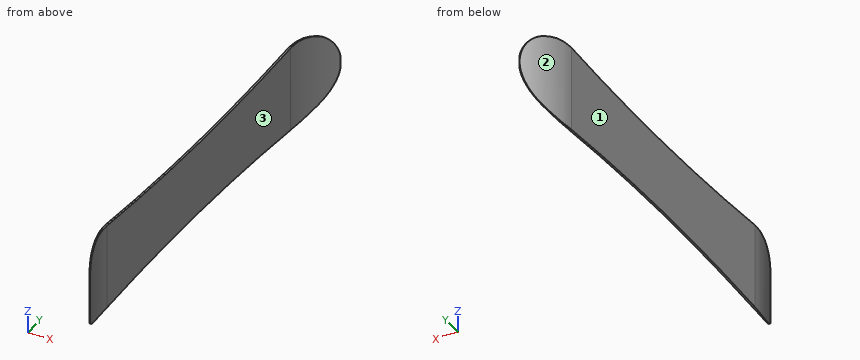
Solid Edge part; units mm, degrees
sketch "Sketch1" plane through (0, 0, 0) normal (1, 0, 0) x (0, 1, 0)
  arc A0 (-585.5098, 151.2) -> (585.5098, 151.2) centre (0, 7528) ccw
  line L0 (585.5098, 151.2) -> (585.5098, -151.2)
  arc A1 (-585.5098, -151.2) -> (585.5098, -151.2) centre (0, -7528) cw
  line L1 (-585.5098, 151.2) -> (-585.5098, -151.2)
extrude "Protrusion1" add sketch "Sketch1" against normal blind 7
sketch "Sketch2" plane through (0, -800, 0) normal (0, 0, -1) x (1, 0, 0)
  arc A0 (59.1552, -1.148) -> (0, -214.4902) centre (414.2845, -214.4902) ccw
  line L0 (0, -214.4902) -> (-7, -214.4902)
  arc A1 (-7, -214.4902) -> (57.4408, -0.1181) centre (446.8281, -234.0406) cw
  line L1 (57.4408, -0.1181) -> (59.1552, -1.148)
extrude "ExtrudedProtrusion_4" add sketch "Sketch2" along normal mid plane 302.4
sketch "Sketch3" plane through (59.1552, 0, 0) normal (1, 0, 0) x (0, 0, 1)
  arc A0 (-128, 717.5098) -> (128, 717.5098) centre (0, 659.2447) cw
  arc A1 (128, 717.5098) -> (151.2, 585.5098) centre (-115.4835, 606.677) cw
  line L0 (265.9453, 585.5098) -> (151.2, 585.5098)
  line L1 (265.9453, 882.5583) -> (265.9453, 585.5098)
  line L2 (-248.3835, 882.5583) -> (265.9453, 882.5583)
  line L3 (-248.3835, 585.5098) -> (-248.3835, 882.5583)
  line L4 (-151.2, 585.5098) -> (-248.3835, 585.5098)
  arc A2 (-151.2, 585.5098) -> (-128, 717.5098) centre (115.4835, 606.677) cw
extrude "Cutout1" cut sketch "Sketch3" against normal through all
mirror "Mirror1" about plane through (0, 0, 0) normal (0, -1, 0) of "ExtrudedProtrusion_4"
sketch "Sketch4" plane through (59.1552, 0, 0) normal (1, 0, 0) x (0, 0, 1)
  line L0 (-268.9862, -585.5098) -> (-151.2, -585.5098)
  arc A0 (-151.2, -585.5098) -> (-128, -717.5098) centre (115.4835, -606.677) ccw
  arc A1 (-128, -717.5098) -> (128, -717.5098) centre (0, -659.2447) ccw
  arc A2 (128, -717.5098) -> (151.2, -585.5098) centre (-115.4835, -606.677) ccw
  line L1 (359.5482, -585.5098) -> (151.2, -585.5098)
  line L2 (359.5482, -919.291) -> (359.5482, -585.5098)
  line L3 (-268.9862, -919.291) -> (359.5482, -919.291)
  line L4 (-268.9862, -585.5098) -> (-268.9862, -919.291)
extrude "Cutout2" cut sketch "Sketch4" against normal through all
Design review of the part built by this model. Coordinates are the model's own, in mm. Face numbers are marked on the shaded views. Give positions to 0.01 mm unless a question says otherwise; leave off trailing zeros. Loops run counter-clockwise (first coordinate to the right, second up) from the corner with the lowest first, then second, coordinate; pieces in that order, holes last. Notation, with made-up numbers: (10, -26.5) -> (20, -26.5) arc R16 ccw to (20, -16.5) -> close; hole circle Ø11 at (81, 23). An arc over 180 degrees is marked (long way). One line per item, written item: value.
Q1. We need section D-D on z = -60.5. Give the boundary of the cut face in (x, y), and give its area (3 significant figures).
Numbers:
outline: (-7, -585.51) arc R454.25 ccw to (49.54, -786.2) -> (51.86, -786.2) arc R414.28 cw to (0, -585.51) -> (0, 585.51) arc R414.28 cw to (51.86, 786.2) -> (49.54, 786.2) arc R454.25 ccw to (-7, 585.51) -> close
area: 9,790 mm^2
Q2. We need section A-A on x = 32. Give the boundary of the cut face in (y, z), and give its area (3 significant figures).
Numbers:
outline: (-751.05, -106.54) arc R140.64 ccw to (-745.17, -111.34) -> (-745.17, 111.34) arc R140.64 ccw to (-751.05, 106.54) -> close; (745.17, -111.34) arc R140.64 ccw to (751.05, -106.54) -> (751.05, 106.54) arc R140.64 ccw to (745.17, 111.34) -> close
area: 2,570 mm^2
Q3. We need section B-B on z = 78.5. Give the boundary of the cut face in (x, y).
Numbers:
outline: (-7, -585.51) arc R454.25 ccw to (44.02, -775.93) -> (46.36, -775.93) arc R414.28 cw to (0, -585.51) -> (0, 585.51) arc R414.28 cw to (46.36, 775.93) -> (44.02, 775.93) arc R454.25 ccw to (-7, 585.51) -> close
Q4. Draft analysis for pull direction Y (two halves, no side actions). For the marked faces 1, 2 and 3, state which applies: pulls with the +Y half, pulls with the -Y half, needs draft (parallel to the pull), parting line crosses it, or undercut.
Numbers:
face 1: needs draft
face 2: pulls with the +Y half
face 3: undercut
Q5. For pin 1 Ø6 at (y, z) = (-398.5, -119) entering from +X; pin 2 Ø1.5 at (x, z) = (49, -60.5) entering from +Y; pin 3 Ø1.5 at (x, z) = (36.5, 107) entering from -Y, all flat-tipped, find the tip position at first contact; note any pin that passes through.
Numbers:
pin 1: stops at x = 0
pin 2: stops at y = 786.39
pin 3: passes through
Q6. We need section C-C on y = 508. Give the boundary of the cut face in (x, z), and give its area (3 significant figures).
Numbers:
outline: (-7, -145.46) -> (0, -145.46) -> (0, 145.46) -> (-7, 145.46) -> close
area: 2,040 mm^2
Q7. For L1, parallel to X at y = 252, z = 71.5; L2, parallel to Y at x = 49, z = 50.5; L3, parallel to Y at x = 42, z = -73.5, list the stretches that pass through material, from the lowest coordinate up.
Numbers:
L1: x = -7 to 0
L2: y = -785.22 to -780.96, 780.96 to 785.22
L3: y = -772.01 to -767.27, 767.27 to 772.01
